Geometry: final body of the model. Coordinates: model frame, mm. Give positions to 0.01 mm unless a question says otherwise; leave off trailing zeros. Write each loop counter-clockwise with the first axis right and the second up, starting at its lowest first coordinate (ties: lowest second). Pieces come first, ordered by that corner, then holes. Notation, with made-up numbers: (2, 65) -> (21, 65) arc R27 cw to (21, 101) -> close; hole circle Ø4 at (-19.75, -27.75). An arc over 180 degrees is marked (long way). Answer in a Markdown table with one row per item. Add a question column.
Item 1: Draft query along Z for faces 1 (the flat face through (-9, -19, 0)), 2 (the cylindrical face through (123.245, -18.783, 26.354)), 3 (the flat face through (-9, 0, 40)). Return one class per face: +Z half, -Z half, draft (parallel to the pull), parting line (faces both ways), or undercut.
Item 2: Material intervals for probe 1 along X at (y, z) = (-11, 25); probe 2 along Z at (x, y) = (69.5, -25); probe 3 along X at (y, z) = (-20.5, 23.5), sorted ascending. Write a range as from..to.
Item 3: First-contact query: P1, Ø4, axis at x = 108.5, y = -16.5, coming from the +Z side; P2, Ø8, axis at x = 7.5, y = -14, coming from the -Z side. Flat tips, straight axial feed; report the tip coordinate or a pass-through.
Item 4: Section query A-A on z = 25.4. Output: boundary loops of the cut face in (x, y), plus the area to 3 significant figures.
Item 5: Section query B-B on y = -3.5. Output: boundary loops of the cut face in (x, z) (3 decimals), plus the area to 3 significant figures.
Item 6: Section query D-D on z = 63.5. Output: boundary loops of the cut face in (x, y), plus the area to 3 significant figures.
Item 7: Section query C-C on x = 120.5. Output: boundary loops of the cut face in (y, z), plus the area to 3 significant figures.
```python
from build123d import *

# Parameters (mm, degrees)
F0_R     = 3.175
F0_R_2   = 6.35
F1_DEPTH = 38.1


with BuildPart() as f1:
    # F0 (on Front) → F1 (new body)
    with BuildSketch(Plane.XZ):
        Polygon((-57.583724, 101.6), (-159.183724, 101.6), (-159.183724, 0), (145.616276, 0), (145.616276, 50.8), align=None)
        with Locations((-133.783724, 25.4)):
            Circle(F0_R, mode=Mode.SUBTRACT)
        with Locations((120.216276, 25.4)):
            Circle(F0_R, mode=Mode.SUBTRACT)
        with Locations((-108.383724, 63.5)):
            Circle(F0_R_2, mode=Mode.SUBTRACT)
    extrude(amount=F1_DEPTH)


solid = f1.part
```
Findings below:
| question | item | result |
|---|---|---|
| 1 | face 1 | -Z half |
| 1 | face 2 | undercut |
| 1 | face 3 | draft |
| 2 | probe 1 | x = -159.18..-136.93, -130.63..117.07, 123.37..145.62 |
| 2 | probe 2 | z = 0..69.83 |
| 2 | probe 3 | x = -159.18..-136.33, -131.24..117.67, 122.76..145.62 |
| 3 | P1 | stops at z = 60.58 |
| 3 | P2 | stops at z = 0 |
| 4 | outline | (-159.18, -38.1) -> (-136.96, -38.1) -> (-136.96, 0) -> (-159.18, 0) -> close; (-130.61, -38.1) -> (117.04, -38.1) -> (117.04, 0) -> (-130.61, 0) -> close; (123.39, -38.1) -> (145.62, -38.1) -> (145.62, 0) -> (123.39, 0) -> close |
| 4 | area | 11,100 mm^2 |
| 5 | outline | (-159.184, 0) -> (145.616, 0) -> (145.616, 50.8) -> (-57.584, 101.6) -> (-159.184, 101.6) -> close; hole circle Ø6.35 at (-133.784, 25.4); hole circle Ø12.7 at (-108.384, 63.5); hole circle Ø6.35 at (120.216, 25.4) |
| 5 | area | 25,600 mm^2 |
| 6 | outline | (-159.18, -38.1) -> (-114.73, -38.1) -> (-114.73, 0) -> (-159.18, 0) -> close; (-102.03, -38.1) -> (94.82, -38.1) -> (94.82, 0) -> (-102.03, 0) -> close |
| 6 | area | 9,190 mm^2 |
| 7 | outline | (-38.1, 0) -> (0, 0) -> (0, 22.24) -> (-38.1, 22.24) -> close; (-38.1, 28.56) -> (0, 28.56) -> (0, 57.08) -> (-38.1, 57.08) -> close |
| 7 | area | 1,930 mm^2 |
